from build123d import *

# Parameters (mm, degrees)
BOSS_EXTRUDE1_DEPTH = 18.25625
SKETCH2_W           = 47.752
SKETCH2_H           = 127
CUT_EXTRUDE1_DEPTH  = 3.81


with BuildPart() as part:
    # Sketch1 → Boss-Extrude1 (new body)
    with BuildSketch(Plane(origin=(0, 0, 0), x_dir=(1, 0, 0), z_dir=(0, 1, 0))):
        Polygon((-489.74375, 381), (-489.74375, 1447.8), (-388.14375, 1447.8), (-388.14375, 381), (489.74375, 381), (489.74375, -381), (-489.74375, -381), align=None)
    extrude(amount=BOSS_EXTRUDE1_DEPTH)

    # Sketch2 → Cut-Extrude1 (cut)
    with BuildSketch(Plane(origin=(0, 18.25625, 0), x_dir=(1, 0, 0), z_dir=(0, 1, 0))):
        with Locations((-465.86775, 1304.527191457)):
            Rectangle(SKETCH2_W, SKETCH2_H)
        with Locations((-465.86775, 533.4)):
            Rectangle(SKETCH2_W, SKETCH2_H)
        with Locations((-465.86775, -237.727191457)):
            Rectangle(SKETCH2_W, SKETCH2_H)
    extrude(amount=-CUT_EXTRUDE1_DEPTH, mode=Mode.SUBTRACT)


solid = part.part
Verification items for the finished model (mm, model axes). A direction names the side the tool comes from. Coordinates: 2 decimals unless noted, no trailing zeros. Order: outer loops, then holes, each group sorted by start corner. A loop starts at its lowest first (then second) coordinate and runs counter-clockwise, first axis right, second up. Notation, with made-up numbers: M 0,74 L 17,74 A25 cw 17,97 Z; hole C -32.75,88 d6. An arc over 180 degrees is marked long. One line per item, written item: value. Start each with the question number.
Item 1: Gauge pin test, flat ends, axial feed: pin 1 (24 mm diameter, centred on x = -458.5, z = -1288, fed in from +Y); pin 2 (3 mm diameter, centred on x = 47, y = 14, fed in from -Z); pin 3 (3 mm diameter, centred on y = 16, z = -519, fed in from -X). Record the tip position at first contact, or that the pin passes through.
Item 2: Access from +Z, -Z, +X, -X, +Y, -Y to the whole of each face (thin tool, end or side, straight path). Record for faces 1 (the flat face through (-466, 14.446, 237)), 2 (the flat face through (7, 0, -140)).
Item 3: Sectioned sample at B-B (z = -876). Enter the section's corners in (x, y), then the cut area to 3 significant figures.
Item 4: Sectioned sample at C-C (x = -163.5). Enter the section's corners in (y, z), then the cut area to 3 significant figures.
Item 5: Sectioned sample at A-A (y = 3.75). Enter the section's corners in (x, z), then the cut area to 3 significant figures.
Item 6: Scan lines: probe 1 along X at (y, z) = (13.5, -997.5); probe 2 along Z at (x, y) = (-37, 13); probe 3 along X at (y, z) = (17, 292.5). Record each from-to range of solid material in increasing order.
Item 7: Mould release check, pull along Z, two halves, no side actions. Record for faces 3 (the flat face through (7, 18.256, -140)), 4 (the flat face through (-466, 14.446, -534)): released by +Z, released by -Z, zero draft, split by the parting line, or undercut.
Conclusion:
1. pin 1: stops at y = 14.45
1. pin 2: stops at z = -381
1. pin 3: stops at x = -441.99
2. face 1: -X, +Y
2. face 2: +Z, -Z, +X, -X, -Y
3. outline: M -489.74,0 L -388.14,0 L -388.14,18.26 L -489.74,18.26 Z
3. area: 1,850 mm^2
4. outline: M 0,-381 L 18.26,-381 L 18.26,381 L 0,381 Z
4. area: 13,900 mm^2
5. outline: M -489.74,-1447.8 L -388.14,-1447.8 L -388.14,-381 L 489.74,-381 L 489.74,381 L -489.74,381 Z
5. area: 855,000 mm^2
6. probe 1: x = -489.74 to -388.14
6. probe 2: z = -381 to 381
6. probe 3: x = -441.99 to 489.74
7. face 3: zero draft
7. face 4: undercut
